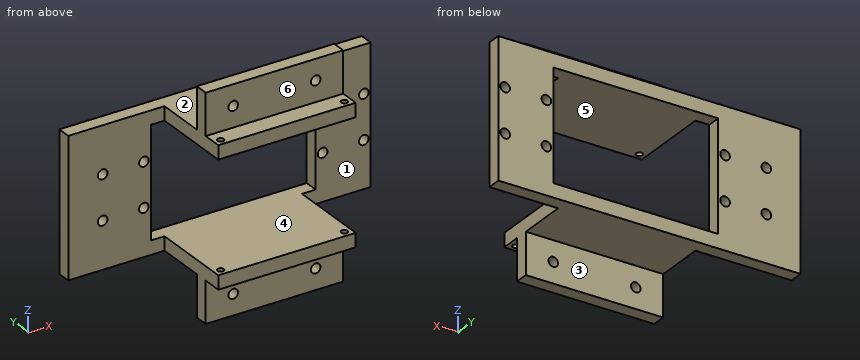
from build123d import *

# Parameters (mm, degrees)
SKETCH3_W               = 100
SKETCH3_H               = 50
SKETCH3_R               = 1.75
BOSS_EXTRUDE1_DEPTH     = 5
CUT_EXTRUDE1_DEPTH      = 57.124860802
CUT_EXTRUDE1_DEPTH_BACK = 57.124860802
SKETCH4_W               = 60
SKETCH4_H               = 40
SKETCH5_W               = 50
SKETCH5_H               = 5
BOSS_EXTRUDE2_DEPTH     = 30
SKETCH6_W               = 50
SKETCH6_H               = 5
BOSS_EXTRUDE3_DEPTH     = 15
SKETCH7_R               = 1.75
CUT_EXTRUDE2_DEPTH      = 69.036754773
SKETCH8_R               = 1.15
CUT_EXTRUDE3_DEPTH      = 88.321245983
SKETCH9_W               = 50
SKETCH9_H               = 5
BOSS_EXTRUDE4_DEPTH     = 10


with BuildPart() as part:
    # Sketch3 → Boss-Extrude1 (new body)
    with BuildSketch(Plane(origin=(0, 0, 0), x_dir=(1, 0, 0), z_dir=(0, 1, 0))):
        Rectangle(SKETCH3_W, SKETCH3_H)
        with Locations(Location((-47.5, 8, 0), (0, 0, 270))):
            Circle(SKETCH3_R, mode=Mode.SUBTRACT)
        with Locations(Location((-32.5, 8, 0), (0, 0, 270))):
            Circle(SKETCH3_R, mode=Mode.SUBTRACT)
        with Locations(Location((-47.5, -8, 0), (0, 0, 270))):
            Circle(SKETCH3_R, mode=Mode.SUBTRACT)
        with Locations(Location((-32.5, -8, 0), (0, 0, 270))):
            Circle(SKETCH3_R, mode=Mode.SUBTRACT)
        with Locations(Location((47.5, -8, 0), (0, 0, 90))):
            Circle(SKETCH3_R, mode=Mode.SUBTRACT)
        with Locations(Location((47.5, 8, 0), (0, 0, 90))):
            Circle(SKETCH3_R, mode=Mode.SUBTRACT)
        with Locations(Location((32.5, 8, 0), (0, 0, 90))):
            Circle(SKETCH3_R, mode=Mode.SUBTRACT)
        with Locations(Location((32.5, -8, 0), (0, 0, 90))):
            Circle(SKETCH3_R, mode=Mode.SUBTRACT)
    extrude(amount=BOSS_EXTRUDE1_DEPTH)

    # Sketch4 → Cut-Extrude1 (cut, two sides: drawn at the far end of the back side and taken through both)
    with BuildSketch(Plane(origin=(0, 5, 0), x_dir=(1, 0, 0), z_dir=(0, 1, 0)).offset(-CUT_EXTRUDE1_DEPTH_BACK)):
        Rectangle(SKETCH4_W, SKETCH4_H)
    extrude(amount=CUT_EXTRUDE1_DEPTH + CUT_EXTRUDE1_DEPTH_BACK, mode=Mode.SUBTRACT)

    # Sketch5 → Boss-Extrude2 (add)
    with BuildSketch(Plane(origin=(0, 0, 0), x_dir=(1, 0, 0), z_dir=(0, 1, 0))):
        with Locations((0, 22.5)):
            Rectangle(SKETCH5_W, SKETCH5_H)
        with Locations((0, -22.5)):
            Rectangle(SKETCH5_W, SKETCH5_H)
    extrude(amount=-BOSS_EXTRUDE2_DEPTH)

    # Sketch6 → Boss-Extrude3 (add)
    with BuildSketch(Plane.XY.offset(25)):
        with Locations((0, -20.5)):
            Rectangle(SKETCH6_W, SKETCH6_H)
    boss_extrude3 = extrude(amount=BOSS_EXTRUDE3_DEPTH)

    # Sketch7 → Cut-Extrude2 (cut, through all)
    with BuildSketch(Plane(origin=(0, -18, 0), x_dir=(1, 0, 0), z_dir=(0, 1, 0))):
        with Locations(Location((-15, -32.5, 0), (0, 0, 270))):
            Circle(SKETCH7_R)
        with Locations(Location((15, -32.5, 0), (0, 0, 270))):
            Circle(SKETCH7_R)
    cut_extrude2 = extrude(amount=-CUT_EXTRUDE2_DEPTH, mode=Mode.SUBTRACT)

    # Mirror1: Boss-Extrude3, Cut-Extrude2 across plane
    add(boss_extrude3.mirror(Plane.XY))
    add(cut_extrude2.mirror(Plane.XY), mode=Mode.SUBTRACT)

    # Sketch8 → Cut-Extrude3 (cut, through all)
    with BuildSketch(Plane.XY.offset(25)):
        with Locations((-22.5, -27.5)):
            Circle(SKETCH8_R)
        with Locations((22.5, -27.5)):
            Circle(SKETCH8_R)
    extrude(amount=-CUT_EXTRUDE3_DEPTH, mode=Mode.SUBTRACT)

    # Sketch9 → Boss-Extrude4 (add)
    with BuildSketch(Plane.ZY.offset(50)):
        with Locations((0, 2.5)):
            Rectangle(SKETCH9_W, SKETCH9_H)
    extrude(amount=BOSS_EXTRUDE4_DEPTH)


solid = part.part
Part model, mm, in its own coordinate system. Face numbers are marked on the shaded views. A direction names the side the tool comes from. Give positions to 0.01 mm unless a question says otherwise; leave off trailing zeros. Loops run counter-clockwise (first coordinate to the right, second up) from the corner with the lowest first, then second, coordinate; pieces in that order, holes last.
(1) Band-saw the part on D-D (z = 18). Write the cut outline in (x, y), and give its area (3 significant figures).
Return value:
outline: (-60, 0) - (-30, 0) - (-30, 5) - (-60, 5) - close; (30, 0) - (50, 0) - (50, 5) - (30, 5) - close
area: 250 mm2
(2) Pull direction X, two halves, no side cores. Call the marked faces 4, 5 and 6: pulls with the +X half, pulls with the -X half, needs draft (parallel to the pull), parting line crosses it, or undercut.
Return value:
face 4: undercut
face 5: undercut
face 6: needs draft
(3) 3-axis set-ups, long thin cutter, end or side, ignore diameter. For the marked faces 1, 2 and 3: which of +Z, -Z, +X, -X, +Y, -Y reach the whole face in a straight line?
Return value:
face 1: +Z, -Z, +X, -Y
face 2: +Z, +X, -X, +Y
face 3: -Z, +X, -X, +Y
(4) Band-saw the part on B-B (z = -8). Write the cut outline in (x, y), and give its area (3 significant figures).
Return value:
outline: (-60, 0) - (-49.25, 0) - (-49.25, 5) - (-60, 5) - close; (-45.75, 0) - (-34.25, 0) - (-34.25, 5) - (-45.75, 5) - close; (-30.75, 0) - (-30, 0) - (-30, 5) - (-30.75, 5) - close; (30, 0) - (30.75, 0) - (30.75, 5) - (30, 5) - close; (34.25, 0) - (45.75, 0) - (45.75, 5) - (34.25, 5) - close; (49.25, 0) - (50, 0) - (50, 5) - (49.25, 5) - close
area: 180 mm2
(5) Band-saw the part on A-A (x = -15). Write the cut outline in (y, z), and give its area (3 significant figures).
Return value:
outline: (-30, -25) - (-23, -25) - (-23, -30.75) - (-18, -30.75) - (-18, -25) - (5, -25) - (5, -20) - (-30, -20) - close; (-30, 20) - (5, 20) - (5, 25) - (-18, 25) - (-18, 30.75) - (-23, 30.75) - (-23, 25) - (-30, 25) - close; (-23, -40) - (-18, -40) - (-18, -34.25) - (-23, -34.25) - close; (-23, 34.25) - (-18, 34.25) - (-18, 40) - (-23, 40) - close
area: 465 mm2
(6) Pin check, flat tips, straight feed: pin 1 (1 mm diameter, centred on x = -47.5, y = -1, fed in from +Z); pin 2 (6 mm diameter, centred on x = 1, y = -16.5, fed in from -Z); pin 3 (6 mm diameter, centred on x = -42, z = 2.5, fed in from -Y); pin 4 (1.5 mm diameter, centred on x = -32.5, y = 0, fed in from -Z). Stop position of each tip, or through.
Return value:
pin 1: passes through
pin 2: stops at z = -40
pin 3: stops at y = 0
pin 4: stops at z = -25
(7) Band-saw the part on C-C (y = 2.5). Count the separate pieces of the cut face and the enclosed holes in it, and give its area (3 significant figures).
Return value:
separate pieces: 1
enclosed holes: 9
area: 3,020 mm2
(8) Drill centre lines: line 1 along X through (y, z) = (-21.85, -32.5); line 2 along X through (y, z) = (1.95, 8); line 3 along Z through (x, y) = (-20.5, -27.5). Where is each one in solid material? Low to high.
Return value:
line 1: x = -25 to -16.75, -13.25 to 13.25, 16.75 to 25
line 2: x = -60 to -49.25, -45.75 to -34.25, -30.75 to -30, 30 to 30.75, 34.25 to 45.75, 49.25 to 50
line 3: z = -25 to -20, 20 to 25
